Geometry: final body of the model. Coordinates: model frame, mm. Face numbers are marked on the shaded views. Give positions to 0.01 mm unless a question says otherwise; leave off trailing zeros. Order: outer loops, then holes, each group sorted by start corner. A loop starts at its lowest first (then second) coordinate and runs counter-clockwise, first axis right, second up. Notation, with made-up numbers: (6, -6) - (54, -6) arc R18 cw to (54, 27) - close; hole circle Ø10 at (-22.75, -11.75). An arc over 180 degrees is marked (long way). Use one line per item in the form item = value.
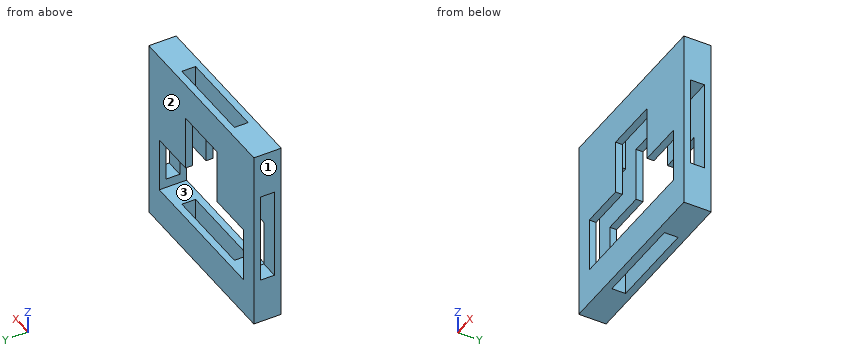
from build123d import *

# Parameters (mm, degrees)
SKETCH1_W           = 20
SKETCH1_H           = 20
BOSS_EXTRUDE1_DEPTH = 3
SKETCH2_W           = 10
SKETCH2_H           = 1.5
CUT_EXTRUDE1_DEPTH  = 21
SKETCH3_W           = 10
SKETCH3_H           = 1.5
CUT_EXTRUDE2_DEPTH  = 21


with BuildPart() as part:
    # Sketch1 → Boss-Extrude1 (new body)
    with BuildSketch(Plane(origin=(0, 0, 0), x_dir=(1, 0, 0), z_dir=(0, 1, 0))):
        Rectangle(SKETCH1_W, SKETCH1_H)
        Polygon((-3, 0), (-8, 0), (-8, 6), (8, 6), (8, 0), (3, 0), (3, -6), (-3, -6), align=None, mode=Mode.SUBTRACT)
    extrude(amount=BOSS_EXTRUDE1_DEPTH)

    # Sketch2 → Cut-Extrude1 (cut, through all)
    with BuildSketch(Plane.XY.offset(10)):
        with Locations((0, 1.5)):
            Rectangle(SKETCH2_W, SKETCH2_H)
    extrude(amount=-CUT_EXTRUDE1_DEPTH, mode=Mode.SUBTRACT)

    # Sketch3 → Cut-Extrude2 (cut, through all)
    with BuildSketch(Plane(origin=(10, 0, 0), x_dir=(0, 0, -1), z_dir=(1, 0, 0))):
        with Locations((0, 1.5)):
            Rectangle(SKETCH3_W, SKETCH3_H)
    extrude(amount=-CUT_EXTRUDE2_DEPTH, mode=Mode.SUBTRACT)


solid = part.part
(1) Pull-direction query (X, two-part tool) for the marked faces 1, 2 and 3; classes: released by +X, released by -X, zero draft, split by the parting line, or undercut.
Computed values:
face_1 = released by -X
face_2 = zero draft
face_3 = undercut
(2) Ray query, line 1 along Z through (x, y) = (-7, 0.45); line 2 along X through (y, z) = (1.15, -5.25); line 3 along Z through (x, y) = (9.25, 1.35). Return the intervals inside material, ascending.
Computed values:
line_1 = -10 to -6, 0 to 10
line_2 = -10 to -8, 8 to 10
line_3 = -10 to -5, 5 to 10
(3) Cut plane A-A on x = -1.75. Output: boundary loops of the cut face in (y, z).
Computed values:
outline = (0, -10) - (0.75, -10) - (0.75, -6) - (0, -6) - close; (0, 6) - (0.75, 6) - (0.75, 10) - (0, 10) - close; (2.25, -10) - (3, -10) - (3, -6) - (2.25, -6) - close; (2.25, 6) - (3, 6) - (3, 10) - (2.25, 10) - close
(4) Cut plane B-B on y = 1.9. Output: boundary loops of the cut face in (x, z).
Computed values:
outline = (-10, -10) - (-5, -10) - (-5, -6) - (-8, -6) - (-8, -5) - (-10, -5) - close; (-10, 5) - (-5, 5) - (-5, 10) - (-10, 10) - close; (5, -10) - (10, -10) - (10, -5) - (8, -5) - (8, -6) - (5, -6) - close; (5, 5) - (10, 5) - (10, 10) - (5, 10) - close
(5) Cut plane C-C on z = -1.25. Output: boundary loops of the cut face in (x, y), plus the area to 3 significant figures.
Computed values:
outline = (-10, 0) - (-8, 0) - (-8, 0.75) - (-10, 0.75) - close; (-10, 2.25) - (-8, 2.25) - (-8, 3) - (-10, 3) - close; (8, 0) - (10, 0) - (10, 0.75) - (8, 0.75) - close; (8, 2.25) - (10, 2.25) - (10, 3) - (8, 3) - close
area = 6.00 mm²
(6) Cut plane D-D on z = 7. Output: boundary loops of the cut face in (x, y), plus the area to 3 significant figures.
Computed values:
outline = (-10, 0) - (10, 0) - (10, 3) - (-10, 3) - close; hole (-5, 0.75) - (5, 0.75) - (5, 2.25) - (-5, 2.25) - close
area = 45.0 mm²
